from build123d import *

# Parameters (mm, degrees)
F0_R      = 37.084
F1_DEPTH  = 3.81
F2_R      = 32.766
F3_DEPTH  = 8.255
F4_R      = 12.192
F5_DEPTH  = 12.065
F6_R      = 25.4
F6_R_2    = 12.192
F7_DEPTH  = 3.302
F8_R      = 14.224
F8_R_2    = 12.192
F9_DEPTH  = 6.604
F11_DEPTH = 12.192
F10_R     = 5.334
F10_R_2   = 2.54
F12_DEPTH = 3.302


with BuildPart() as f1:
    # F0 (on Top) → F1 (new body)
    with BuildSketch(Plane.XY):
        with Locations((44.6336865425, -8.3147734404)):
            Circle(F0_R)
    extrude(amount=F1_DEPTH)

    # F2 (on face) → F3 (join)
    with BuildSketch(Plane.XY.offset(3.81)):
        with Locations((44.6336865425, -8.3147734404)):
            Circle(F2_R)
    extrude(amount=F3_DEPTH)

    # F4 (on face) → F5 (cut)
    with BuildSketch(Plane.XY.offset(12.065)):
        with Locations((44.6336865425, -8.3147734404)):
            Circle(F4_R)
    extrude(amount=-F5_DEPTH, mode=Mode.SUBTRACT)

    # F6 (on face) → F7 (cut)
    with BuildSketch(Plane(origin=(0, 0, 0), x_dir=(1, 0, 0), z_dir=(0, 0, -1))):
        with Locations((44.6336865425, 8.3147734404)):
            Circle(F6_R)
        with Locations((44.6336865425, 8.3147734404)):
            Circle(F6_R_2, mode=Mode.SUBTRACT)
    extrude(amount=-F7_DEPTH, mode=Mode.SUBTRACT)

    # F8 (on face) → F9 (cut)
    with BuildSketch(Plane(origin=(0, 0, 3.302), x_dir=(1, 0, 0), z_dir=(0, 0, -1))):
        with Locations((44.6336865425, 8.3147734404)):
            Circle(F8_R)
        with Locations((44.6336865425, 8.3147734404)):
            Circle(F8_R_2, mode=Mode.SUBTRACT)
    extrude(amount=-F9_DEPTH, mode=Mode.SUBTRACT)

    # F10 (on face) → F11 (cut)
    with BuildSketch(Plane(origin=(0, 0, 0), x_dir=(1, 0, 0), z_dir=(0, 0, -1))):
        with BuildLine():
            ThreePointArc((26.4725169512, -3.5816526428), (24.4962514712, -1.1050009937), (21.6427505016, -2.4823030141))
            ThreePointArc((21.6427505016, -2.4823030141), (22.6111657007, -4.3409989885), (23.7295214672, -6.1135280018))
            ThreePointArc((23.7295214672, -6.1135280018), (25.6553041509, -5.4480942478), (26.4725169512, -3.5816526428))
        make_face()
        with BuildLine():
            ThreePointArc((23.7295214672, -6.1135280018), (22.6111657007, -4.3409989885), (21.6427505016, -2.4823030141))
            ThreePointArc((21.6427505016, -2.4823030141), (21.730264867, -4.8472298857), (23.7295214672, -6.1135280018))
        make_face()
        with BuildLine():
            ThreePointArc((26.5204945446, 20.2942991529), (25.7070287844, 22.1572751374), (23.7876760259, 22.8269698814))
            ThreePointArc((23.7876760259, 22.8269698814), (22.6622056937, 21.0589497303), (21.6863284225, 19.2041607194))
            ThreePointArc((21.6863284225, 19.2041607194), (24.5392512224, 17.8165197085), (26.5204945446, 20.2942991529))
        make_face()
        with BuildLine():
            ThreePointArc((21.6863284225, 19.2041607194), (22.6622056937, 21.0589497303), (23.7876760259, 22.8269698814))
            ThreePointArc((23.7876760259, 22.8269698814), (21.7833464597, 21.5687167819), (21.6863284225, 19.2041607194))
        make_face()
        with BuildLine():
            ThreePointArc((47.2216641359, 32.1907252361), (47.1083746403, 32.9408426453), (46.7786120668, 33.6240463358))
            ThreePointArc((46.7786120668, 33.6240463358), (44.6847265355, 33.7147221592), (42.5904934978, 33.6324621615))
            ThreePointArc((42.5904934978, 33.6324621615), (43.9266718912, 29.7655269534), (47.2216641359, 32.1907252361))
        make_face()
        with BuildLine():
            ThreePointArc((42.5904934978, 33.6324621615), (44.6847265355, 33.7147221592), (46.7786120668, 33.6240463358))
            ThreePointArc((46.7786120668, 33.6240463358), (44.6867681352, 34.7307201079), (42.5904934978, 33.6324621615))
        make_face()
        with BuildLine():
            ThreePointArc((67.6246225834, 19.1118498948), (66.6562073843, 20.9705458693), (65.5378516178, 22.7430748825))
            ThreePointArc((65.5378516178, 22.7430748825), (63.1326040496, 18.9456222806), (67.6246225834, 19.1118498948))
        make_face()
        with BuildLine():
            ThreePointArc((67.6246225834, 19.1118498948), (67.8115077829, 19.6474650036), (67.8748561338, 20.2111995235))
            ThreePointArc((67.8748561338, 20.2111995235), (67.2012977387, 21.9339867232), (65.5378516178, 22.7430748825))
            ThreePointArc((65.5378516178, 22.7430748825), (66.6562073843, 20.9705458693), (67.6246225834, 19.1118498948))
        make_face()
        with BuildLine():
            ThreePointArc((67.8268785404, -3.6647522722), (67.7646579848, -3.1059955944), (67.5810446625, -2.5746138386))
            ThreePointArc((67.5810446625, -2.5746138386), (66.6051673914, -4.4294028496), (65.4796970591, -6.1974230006))
            ThreePointArc((65.4796970591, -6.1974230006), (67.1498545249, -5.391286512), (67.8268785404, -3.6647522722))
        make_face()
        with BuildLine():
            ThreePointArc((65.4796970591, -6.1974230006), (66.6051673914, -4.4294028496), (67.5810446625, -2.5746138386))
            ThreePointArc((67.5810446625, -2.5746138386), (63.0897304555, -2.3903346432), (65.4796970591, -6.1974230006))
        make_face()
        with BuildLine():
            ThreePointArc((42.4887610182, -16.9944994551), (44.5806049498, -18.1011732272), (46.6768795873, -17.0029152808))
            ThreePointArc((46.6768795873, -17.0029152808), (44.5826465496, -17.0851752785), (42.4887610182, -16.9944994551))
        make_face()
        with BuildLine():
            ThreePointArc((42.4887610182, -16.9944994551), (44.5826465496, -17.0851752785), (46.6768795873, -17.0029152808))
            ThreePointArc((46.6768795873, -17.0029152808), (47.0109072318, -16.3161706001), (47.1257089491, -15.5611783553))
            ThreePointArc((47.1257089491, -15.5611783553), (43.8355915399, -13.1344678509), (42.4887610182, -16.9944994551))
        make_face()
    extrude(amount=-F11_DEPTH, mode=Mode.SUBTRACT)

    # F10 (on face) → F12 (cut)
    with BuildSketch(Plane(origin=(0, 0, 0), x_dir=(1, 0, 0), z_dir=(0, 0, -1))):
        with Locations((44.6816641359, 32.1907252361)):
            Circle(F10_R)
        with Locations((44.6816641359, 32.1907252361)):
            Circle(F10_R_2, mode=Mode.SUBTRACT)
        with Locations((65.3348561338, 20.2111995235)):
            Circle(F10_R)
        with Locations((65.3348561338, 20.2111995235)):
            Circle(F10_R_2, mode=Mode.SUBTRACT)
        with Locations((65.2868785404, -3.6647522722)):
            Circle(F10_R)
        with Locations((65.2868785404, -3.6647522722)):
            Circle(F10_R_2, mode=Mode.SUBTRACT)
        with Locations((44.5857089491, -15.5611783553)):
            Circle(F10_R)
        with Locations((44.5857089491, -15.5611783553)):
            Circle(F10_R_2, mode=Mode.SUBTRACT)
        with Locations((23.9325169512, -3.5816526428)):
            Circle(F10_R)
        with Locations((23.9325169512, -3.5816526428)):
            Circle(F10_R_2, mode=Mode.SUBTRACT)
        with Locations((23.9804945446, 20.2942991529)):
            Circle(F10_R)
        with Locations((23.9804945446, 20.2942991529)):
            Circle(F10_R_2, mode=Mode.SUBTRACT)
    extrude(amount=-F12_DEPTH, mode=Mode.SUBTRACT)


solid = f1.part
Part model, mm, in its own coordinate system. A direction names the side the tool comes from. Coordinates: 2 decimals unless noted, no trailing zeros. Loops run counter-clockwise (first coordinate to the right, second up) from the corner with the lowest first, then second, coordinate; pieces in that order, holes last. Notation, with made-up numbers: M 16,29 L 35,29 A7 ccw 35,39 Z; hole C 36.25,33 d2. An arc over 180 degrees is marked long. Use a Markdown table: item, result. Add a question column.
Q1. Pin check, flat tips, straight feed: P1, Ø6, axis at x = 36.5, z = 2.5, coming from the -Y side; P2, Ø5, axis at x = 26.5, z = 1.5, coming from the -Y side; P3, Ø6, axis at x = 63, y = -11.5, coming from the -Z side. Stop position of each tip, or through.
Q2. Mould opens along Y. For faces 1 (the cylindrical face through (18.63, -28.25, 7.88)), 2 (the flat face through (52, -33, 0)), 3 (the cylindrical face through (44.471, 20.894, 1.628)) say: +Y half, -Y half, draft (parallel to the pull), parting line (faces both ways), or undercut.
Q3. Cut at C-C (z = 1). Write the cut outline in (x, y), and give its area (3 significant figures).
Q4. Cut at B-B (z = 7). Write the cut outline in (x, y), and give its area (3 significant figures).
Q5. Cut at A-A (x = 64.5). Write the cut outline in (y, z) (3 decimals), and give its area (3 significant figures).
Q6. Which spindle directions (+Z, -Z, +X, -X, +Y, -Y) get a long thin tool onto all of the face, cutting with end or side? Do faces 4 (the cylindrical face through (69.85, 6.43, 1.63)), 5 (the cylindrical face through (78.89, -22.52, 1.88)), 6 (the flat face through (58.2, -38.4, 3.81)). Say none if no direction does.
Q7. Probe L1, parallel to Y at x = 23, z = 8.5; L2, parallel to X at y = -8, z = 0.5; L3, parallel to Z at x = 20, y = -22 (3 decimals). List the from-to ranges inside material, lowest first.
Q8. Cut at D-D (y = 10). Write the cut outline in (x, z) (1 decimal), and give its area (3 significant figures).
Worked out:
| question | item | result |
|---|---|---|
| 1 | P1 | stops at y = -45.04 |
| 1 | P2 | stops at y = -41.94 |
| 1 | P3 | stops at z = 3.3 |
| 2 | face 1 | parting line |
| 2 | face 2 | draft |
| 2 | face 3 | undercut |
| 3 | outline | C 44.63,-8.31 d74.17; hole M 20.47,-0.48 A25.4 ccw 20.5,-16.25 A5.33 ccw 25.77,-25.32 A25.4 ccw 39.44,-33.18 A5.33 ccw 49.93,-33.16 A25.4 ccw 63.57,-25.24 A5.33 ccw 68.79,-16.15 A25.4 ccw 68.76,-0.38 A5.33 ccw 63.5,8.69 A25.4 ccw 49.83,16.55 A5.33 ccw 39.34,16.53 A25.4 ccw 25.7,8.61 A5.33 ccw Z |
| 3 | area | 2,110 mm2 |
| 4 | outline | C 44.63,-8.31 d65.53; hole C 23.93,3.58 d5.08; hole C 23.98,-20.29 d5.08; hole C 44.63,-8.31 d28.45; hole C 44.59,15.56 d5.08; hole C 44.68,-32.19 d5.08; hole C 65.29,3.66 d5.08; hole C 65.33,-20.21 d5.08 |
| 4 | area | 2,620 mm2 |
| 5 | outline | M -39.629,0 L -25.479,0 L -25.479,3.302 L -22.61,3.302 L -22.61,12.065 L -34.371,12.065 L -34.371,3.81 L -39.629,3.81 Z; M -17.812,3.302 L 1.25,3.302 L 1.25,12.065 L -17.812,12.065 Z; M 6.08,3.302 L 8.94,3.302 L 8.94,0 L 22.999,0 L 22.999,3.81 L 17.742,3.81 L 17.742,12.065 L 6.08,12.065 Z |
| 5 | area | 471 mm2 |
| 6 | face 4 | -Z |
| 6 | face 5 | +Z, -Z |
| 6 | face 6 | +Z |
| 7 | L1 | y = -32.92 to -22.64, -17.95 to 1.22, 5.94 to 16.29 |
| 7 | L2 | x = 7.55 to 19.24, 70.03 to 81.72 |
| 7 | L3 | z = 3.302 to 12.065 |
| 8 | outline | M 12.4,0 L 27,0 L 27,3.3 L 62.2,3.3 L 62.2,0 L 76.9,0 L 76.9,3.8 L 71.8,3.8 L 71.8,12.1 L 17.5,12.1 L 17.5,3.8 L 12.4,3.8 Z |
| 8 | area | 578 mm2 |
